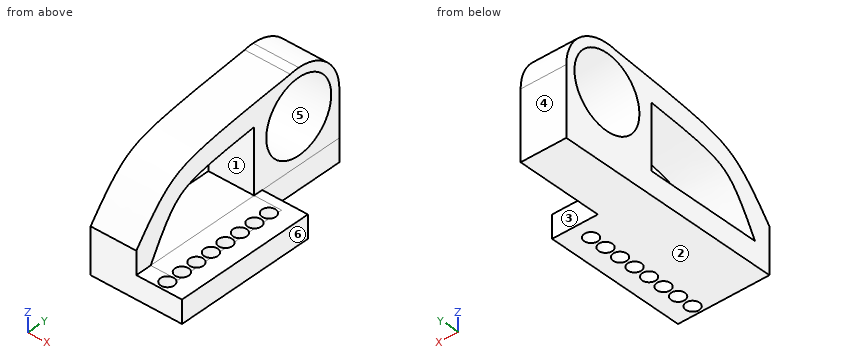
Autodesk Fusion 360 part; units mm, degrees
sketch "Sketch1" plane through (0, 0, 0) normal (0, 0, 1) x (1, 0, 0)
  line L0 (0, 0) -> (20, 0)
  line L1 (20, 0) -> (20, 50)
  line L2 (20, 50) -> (0, 50)
  line L3 (0, 50) -> (0, 0)
  dimension "d1" = 50
extrude "Extrude1" add sketch "Sketch1" along normal blind 30
sketch "Sketch2" plane through (0, 0, 0) normal (0, -1, 0) x (1, 0, 0)
  line L0 (0, 0) -> (20, 0)
  line L1 (20, 0) -> (20, 30)
  line L2 (20, 30) -> (0, 30)
  line L3 (0, 30) -> (0, 0)
  line L4 (0, 30) -> (10, 30)
  line L5 (20, 0) -> (20, 5)
  line L6 (20, 5) -> (10, 5)
  line L7 (10, 5) -> (10, 30)
  dimension "d4" = 5
extrude "Extrude2" cut sketch "Sketch2" against normal blind 70 contours L1 L2 L6 L7
sketch "Sketch3" plane through (0, 0, 0) normal (-1, 0, 0) x (0, -1, 0)
  line L0 (-50, 0) -> (0, 0)
  line L1 (0, 0) -> (0, 30)
  line L2 (0, 30) -> (-50, 30)
  line L3 (-50, 30) -> (-50, 0)
  line L4 (-50, 15) -> (-40, 15)
  line L5 (-40, 15) -> (-40, 30)
  circle A0 centre (-40, 15) radius 8
  dimension "d7" = 16
extrude "Extrude3" cut sketch "Sketch3" against normal blind 15 contours L4 L5 A0 | L4 L5 A0
sketch "Sketch4" plane through (0, 0, 5) normal (0, 0, 1) x (-1, 0, 0)
  line L0 (-20, -50) -> (-10, -50)
  line L1 (-10, -50) -> (-10, 0)
  line L2 (-10, 0) -> (-20, 0)
  line L3 (-20, 0) -> (-20, -50)
  circle A0 centre (-15, -45) radius 0.25
  line L4 (-10, -30) -> (-20, -30)
  circle A1 centre (-15, -27.0301) radius 1.5
  circle A2 centre (-15, -23.4587) radius 1.5
  circle A3 centre (-15, -19.8873) radius 1.5
  circle A4 centre (-15, -16.3158) radius 1.5
  circle A5 centre (-15, -12.7444) radius 1.5
  circle A6 centre (-15, -9.173) radius 1.5
  circle A7 centre (-15, -5.6015) radius 1.5
  circle A8 centre (-15, -2.0301) radius 1.5
  dimension "d11" = 3
  dimension "d14" = 0
  dimension "d15" = 25
extrude "Extrude4" cut sketch "Sketch4" against normal blind 15 contours A1 | A2 | A3 | A4 | A5 | A6 | A7 | A8
sketch "Sketch5" plane through (0, 0, 0) normal (-1, 0, 0) x (0, -1, 0)
  circle A0 centre (-40, 15) radius 8
  line L0 (-50, 0) -> (0, 0)
  line L1 (0, 0) -> (0, 30)
  line L2 (0, 30) -> (-50, 30)
  line L3 (-50, 30) -> (-50, 0)
  circle A1 centre (-40, 15) radius 10
  spline S0 degree 2 poles (-40, 25) (-9.0379, 21.8056) (0, 10) knots 0 0 0 4.447549 4.447549 4.447549 weights 1 3 1
extrude "Extrude5" cut sketch "Sketch5" against normal blind 60 contours L1 L2 L3 A1 S0
sketch "Sketch6" plane through (0, 0, 0) normal (-1, 0, 0) x (0, -1, 0)
  arc A0 (-37.945, 24.7866) -> (-50, 15) centre (-40, 15) ccw
  line L0 (-50, 15) -> (-50, 0)
  line L1 (-50, 0) -> (0, 0)
  line L2 (0, 0) -> (0, 10)
  spline S0 degree 2 poles (0, 10) (-9.0024, 21.7593) (-37.945, 24.7866) knots -4.447549 -4.447549 -4.447549 -0.051947 -0.051947 -0.051947 weights 1 2.97664 1.046174
  circle A1 centre (-40, 15) radius 8
  line L3 (-3, 4) -> (-4, 4)
  line L4 (-4, 4) -> (-29, 4)
  line L5 (-29, 4) -> (-29, 19)
  spline S1 degree 2 poles (-29, 19) (-10, 17) (-3, 4) knots 0 0 0 3.222354 3.222354 3.222354 weights 1 3 1
  line L6 (-3.5416, 5) -> (-29, 5)
extrude "Extrude6" cut sketch "Sketch6" against normal blind 16 contours L5 S1 L6
sketch "Sketch7" plane through (0, 0, 5) normal (0, 0, 1) x (-1, 0, 0)
  circle A0 centre (-15, -9.173) radius 1.5
  circle A1 centre (-15, -5.6015) radius 1.5
  circle A2 centre (-15, -12.7444) radius 1.5
  circle A3 centre (-15, -16.3158) radius 1.5
  line L0 (-10, -3.5416) -> (-10, 0)
  line L1 (-10, 0) -> (-20, 0)
  line L2 (-20, 0) -> (-20, -50)
  line L3 (-20, -50) -> (-10, -50)
  line L4 (-10, -50) -> (-10, -29)
  line L5 (-10, -29) -> (0, -29)
  line L6 (0, -29) -> (0, -3.5416)
  line L7 (0, -3.5416) -> (-10, -3.5416)
  circle A4 centre (-15, -19.8873) radius 1.5
  circle A5 centre (-15, -27.0301) radius 1.5
  circle A6 centre (-15, -23.4587) radius 1.5
  circle A7 centre (-15, -2.0301) radius 1.5
  line L8 (-10, -50) -> (-10, -31)
  line L9 (-20, -31) -> (-10, -31)
  line L10 (-20, -31) -> (-20, -50)
  line L11 (-10, -50) -> (-20, -50)
extrude "Extrude7" cut sketch "Sketch7" against normal blind 15 contours L2 L3 L4 L8 L9 L10 L11
Check sheet for the modelled part. Datum: model origin and axes. Units: mm. Face numbers are marked on the shaded views. A direction names the side the tool comes from. Coordinates: 2 decimals unless noted, no trailing zeros. Order: outer loops, then holes, each group sorted by start corner. A loop starts at its lowest first (then second) coordinate and runs counter-clockwise, first axis right, second up. Notation, with made-up numbers: M 5.5,54.5 L 53.5,54.5 A14 ccw 53.5,78.5 Z; hole C -27,-13.75 d3. An arc over 180 degrees is marked long. One line per question, with ' | ' between items. Start each with the question number.
Item 1: Gauge pin test, flat ends, axial feed: P1, Ø10, axis at y = 31.5, z = 15, coming from the +X side; P2, Ø2.5, axis at x = 15, y = 19.89, coming from the +Z side; P3, Ø5, axis at x = 13.5, y = 16.5, coming from the +Z side; P4, Ø12, axis at x = 7, z = 22.5, coming from the +Y side. Record the tip position at first contact, or that the pin passes through.
Item 2: Sectioned sample at C-C on x = 17.5. Record the cut outline in (y, z), and give its area (3 significant figures).
Item 3: Sectioned sample at B-B on x = 15. Count the separate pieces of the cut face and the enclosed holes in it, and give its area (3 significant figures).
Item 4: Material ranges on line 1 (Z direction, x = 7.5, y = 40); line 2 (X direction, y = 9.5, z = 18.5); line 3 (Z direction, x = 3.5, y = 41), recorded low to high.
Item 5: Access from +Z, -Z, +X, -X, +Y, -Y to the whole of each face (thin tool, end or side, straight path). Record for the marked faces 1, 2 and 3.
Item 6: Sectioned sample at A-A on y = 45. Record the cut outline in (x, z) (3 decimals), and give its area (3 significant figures).
Item 7: Mould release check, pull along Y, two halves, no side actions. Record for the marked faces 4, 5 and 6: pulls with the +Y half, pulls with the -Y half, needs draft (parallel to the pull), parting line crosses it, or undercut.
Answer below:
1) P1: stops at x = 10 | P2: passes through | P3: stops at z = 5 | P4: stops at y = 49.89
2) outline: M 0,0 L 31,0 L 31,5 L 0,5 Z | area: 155 mm^2
3) separate pieces: 9 | enclosed holes: 0 | area: 35.0 mm^2
4) line 1: z = 0 to 7, 23 to 25 | line 2: x = 0 to 10 | line 3: z = 0 to 7.06, 22.94 to 24.95
5) face 1: +X, -X | face 2: -Z, +X, -X, +Y, -Y | face 3: +Z, -Z, +X, +Y
6) outline: M 0,0 L 10,0 L 10,8.755 L 0,8.755 Z; M 0,21.245 L 10,21.245 L 10,23.66 L 0,23.66 Z | area: 112 mm^2
7) face 4: pulls with the +Y half | face 5: undercut | face 6: needs draft
